from build123d import *

# Parameters (mm, degrees)
SKETCH_1_W          = 43
SKETCH_1_H          = 22
EXTRUDE_2_DEPTH     = 10
SKETCH_3_W          = 39
SKETCH_3_H          = 18
CUT_EXTRUDE_1_DEPTH = 9.2
SKETCH_4_W          = 3.2
SKETCH_4_H          = 1.6
CUT_EXTRUDE_2_DEPTH = 2


with BuildPart() as part:
    # Эскиз1 → Бобышка-Вытянуть2 (new body)
    with BuildSketch(Plane(origin=(0, 0, 0), x_dir=(1, 0, 0), z_dir=(0, 1, 0))):
        Rectangle(SKETCH_1_W, SKETCH_1_H)
    extrude(amount=EXTRUDE_2_DEPTH)

    # Эскиз3 → Вырез-Вытянуть1 (cut)
    with BuildSketch(Plane(origin=(0, 10, 0), x_dir=(1, 0, 0), z_dir=(0, 1, 0))):
        Rectangle(SKETCH_3_W, SKETCH_3_H)
    extrude(amount=-CUT_EXTRUDE_1_DEPTH, mode=Mode.SUBTRACT)

    # Эскиз4 → Вырез-Вытянуть2 (cut)
    with BuildSketch(Plane(origin=(0, 0, -11), x_dir=(-1, 0, 0), z_dir=(0, 0, -1))):
        with Locations((-17.9, 2.8)):
            Rectangle(SKETCH_4_W, SKETCH_4_H)
    extrude(amount=-CUT_EXTRUDE_2_DEPTH, mode=Mode.SUBTRACT)


solid = part.part
CAD build for the part. Positions are in the model's coordinates, mm. A direction names the side the tool comes from. Round coordinates to 2 decimals unless told otherwise and drop trailing zeros. Loops run counter-clockwise (first coordinate to the right, second up) from the corner with the lowest first, then second, coordinate; pieces in that order, holes last.
(1) Cut at D-D (x = -4). Give the cut face in (y, z), plus the area to 3 significant figures.
(2) Two-plate mould, pull along X, no slides. Class faces 1 (the flat face through (21.5, 5, 0)), 2 (the flat face through (0, 10, -10)), 3 (the flat face through (-19.5, 5, 0)): +X half, -X half, draft (parallel to the pull), parting line (faces both ways), or undercut.
(3) Which spindle directions (+Z, -Z, +X, -X, +Y, -Y) get a long thin tool onto all of the face, cutting with end or side? Do faces 4 (the flat face through (0, 5, 11)), 5 (the flat face through (18, 3.6, -10)), 6 (the flat face through (0, 5, 9)). Say none if no direction does.
(4) Cut at C-C (y = 2.5). Give the cut face in (x, z).
(5) Cut at A-A (y = 8.5). Give the cut face in (x, z), plus the area to 3 significant figures.
(6) Cut at B-B (z = -6.5). Give the cut face in (x, y), plus the area to 3 significant figures.
(7) Wall check: line 1 along Z through (x, y) = (-5, 8); line 2 along X through (y, z) = (2, -7.5); line 3 along Y through (x, z) = (2, 5.25). Give the ranges that are in metal, low to high.
(8) Drop a flat-ended pin along its axis: pin 1 (3 mm diameter, centred on x = 16, z = 0.5, fed in from +Y). Give the stop position or say it passes through.
Findings below:
1. outline: (0, -11) - (10, -11) - (10, -9) - (0.8, -9) - (0.8, 9) - (10, 9) - (10, 11) - (0, 11) - close
1. area: 54.4 mm2
2. face 1: +X half
2. face 2: draft
2. face 3: undercut
3. face 4: +Z, +X, -X, +Y, -Y
3. face 5: -Z
3. face 6: +Y
4. outline: (-21.5, -11) - (16.3, -11) - (16.3, -9) - (-19.5, -9) - (-19.5, 9) - (19.5, 9) - (19.5, -11) - (21.5, -11) - (21.5, 11) - (-21.5, 11) - close
5. outline: (-21.5, -11) - (21.5, -11) - (21.5, 11) - (-21.5, 11) - close; hole (-19.5, -9) - (19.5, -9) - (19.5, 9) - (-19.5, 9) - close
5. area: 244 mm2
6. outline: (-21.5, 0) - (21.5, 0) - (21.5, 10) - (19.5, 10) - (19.5, 0.8) - (-19.5, 0.8) - (-19.5, 10) - (-21.5, 10) - close
6. area: 71.2 mm2
7. line 1: z = -11 to -9, 9 to 11
7. line 2: x = -21.5 to -19.5, 19.5 to 21.5
7. line 3: y = 0 to 0.8
8. pin 1: stops at y = 0.8
